For this review, take the finished solid that the model builds, in its own axes (mm). Give positions to 0.01 mm unless a question says otherwise; leave off trailing zeros.
Item 1: For P1, Ø10, axis at y = 3, z = -6.5, coming from the -X side; P2, Ø8, axis at x = 10, y = 9, coming from the +Z side; P3, Ø6, axis at y = 10, z = 4.5, coming from the +X side, all flat-tipped, find the tip position at first contact; note any pin that passes through.
Item 2: The part is to be moulded in two halves that separate along Z. For faces 1 (the conical face through (13.383, 9.126, -13.092)), 2 (the flat face through (0, 18, 0)), 3 (the conical face through (13.092, 9.126, 13.383)), say which applies: released by +Z, released by -Z, zero draft, split by the parting line, or undercut.
Item 3: For probe 1 along Y at (x, z) = (-6.5, -21); probe 2 along Z at (x, y) = (3.5, 4); probe 3 along Y at (x, z) = (20.5, 11), list the stretches that pass through material, from the lowest coordinate up.
```python
from build123d import *

# Parameters (mm, degrees)
SKETCH1_W           = 50
SKETCH1_H           = 50
BOSS_EXTRUDE1_DEPTH = 18
FILLET1_R           = 25
CHAMFER1_SIZE       = 11.547005384
CHAMFER1_SIZE_2     = 20


# Some blends are built 0.0001 mm under size
with BuildPart() as part:
    # Sketch1 → Boss-Extrude1 (new body)
    with BuildSketch(Plane(origin=(0, 0, 0), x_dir=(1, 0, 0), z_dir=(0, 1, 0))):
        Rectangle(SKETCH1_W, SKETCH1_H)
    extrude(amount=BOSS_EXTRUDE1_DEPTH)

    # Fillet1
    fillet1_edges = [part.edges().sort_by_distance(p)[0] for p in [
        (-25, 9, -25),
        (25, 9, -25),
        (25, 9, 25),
        (-25, 9, 25),
    ]]
    fillet(fillet1_edges, radius=FILLET1_R - 0.0001)  # a hair under: the kernel refuses the full size

    # Chamfer1
    # the kernel refuses this chamfer: 20, 11.547005384 mm, written as the material it takes off along each edge
    with BuildSketch(Plane(origin=(0.0001, 0, 0.0001), x_dir=(0, 0, 1), z_dir=(-1, 0, 0))) as chamfer1_piece_1:
        Polygon((24.9999 - CHAMFER1_SIZE, 0), (24.9999, CHAMFER1_SIZE_2), (24.9999, 0), align=None)
    revolve(axis=Axis((0.0001, 0, 0.0001), (0, 1, 0)), revolution_arc=90, mode=Mode.SUBTRACT)
    with BuildSketch(Plane(origin=(0.0001, 0, -0.0001), x_dir=(1, 0, 0), z_dir=(0, 0, 1))) as chamfer1_piece_2:
        Polygon((24.9999 - CHAMFER1_SIZE, 0), (24.9999, CHAMFER1_SIZE_2), (24.9999, 0), align=None)
    revolve(axis=Axis((0.0001, 0, -0.0001), (0, 1, 0)), revolution_arc=90, mode=Mode.SUBTRACT)
    with BuildSketch(Plane(origin=(-0.0001, 0, -0.0001), x_dir=(0, 0, -1), z_dir=(1, 0, 0))) as chamfer1_piece_3:
        Polygon((24.9999 - CHAMFER1_SIZE, 0), (24.9999, CHAMFER1_SIZE_2), (24.9999, 0), align=None)
    revolve(axis=Axis((-0.0001, 0, -0.0001), (0, 1, 0)), revolution_arc=90, mode=Mode.SUBTRACT)
    with BuildSketch(Plane(origin=(-0.0001, 0, 0.0001), x_dir=(0, 0, 1), z_dir=(1, 0, 0))) as chamfer1_piece_4:
        Polygon((24.9999 - CHAMFER1_SIZE, 0), (24.9999, -CHAMFER1_SIZE_2), (24.9999, 0), align=None)
    revolve(axis=Axis((-0.0001, 0, 0.0001), (0, -1, 0)), revolution_arc=90, mode=Mode.SUBTRACT)
    with BuildSketch(Plane(origin=(-0.0001, 0, 25), x_dir=(0, 0.9998132206222079, 0.019326765612700806), z_dir=(1, 0, 0))) as chamfer1_piece_5:
        Polygon((CHAMFER1_SIZE_2 * 0.999813220622, -CHAMFER1_SIZE_2 * 0.0193267656127), (-CHAMFER1_SIZE * 0.0193267656124, -CHAMFER1_SIZE * 0.999813220604), (0, 0), align=None)
    extrude(amount=0.0002, mode=Mode.SUBTRACT)
    with BuildSketch(Plane(origin=(-25, 0, -0.0001), x_dir=(0.9983227437537926, -0.05789386240267081, 0), z_dir=(0, 0, 1)), Plane(origin=(0.0001, 0, -25), x_dir=(0, -0.05789386240267081, 0.9983227437537926), z_dir=(-1, 0, 0)), Plane(origin=(25, 0, 0.0001), x_dir=(-0.9983227437537926, -0.05789386240267081, 0), z_dir=(0, 0, -1))) as chamfer1_piece_6:
        Polygon((CHAMFER1_SIZE * 0.998322743736, CHAMFER1_SIZE * 0.0578938624016), (-CHAMFER1_SIZE_2 * 0.0578938624027, CHAMFER1_SIZE_2 * 0.998322743754), (0, 0), align=None)
    extrude(amount=0.0002, mode=Mode.SUBTRACT)


solid = part.part
```
Resolved:
1. P1: stops at x = -17.25
1. P2: stops at z = 19.04
1. P3: stops at x = 20.57
2. face 1: released by -Z
2. face 2: zero draft
2. face 3: released by +Z
3. probe 1: y = 14.77 to 18
3. probe 2: z = -15.37 to 15.37
3. probe 3: y = 16.99 to 18
